Autodesk Fusion 360 part; units mm, degrees
sketch "Sketch1" plane through (0, 0, 0) normal (0, 1, 0) x (1, 0, 0)
  line L0 (-21.4929, -3.9767) -> (-14.25, -3.9767)
  arc A0 (14.25, 0) -> (-14.25, 0) centre (0, 0) ccw
  line L1 (-21.4929, -3.9767) -> (-21.4929, 15.251)
  line L2 (21.5026, 15.251) -> (-21.4929, 15.251)
  circle A1 centre (-17.5048, 0.0114) radius 2.1
  line L3 (21.5026, -4.0254) -> (14.25, -4.0217)
  circle A2 centre (17.4952, -0.0012) radius 2.1
  line L4 (21.5026, -4.0254) -> (21.5026, 15.251)
  line L5 (-21.4929, 11.251) -> (-8.7451, 11.251)
  line L6 (8.7451, 11.251) -> (21.5026, 11.251)
  line L7 (-14.25, -3.9767) -> (-14.25, 0)
  line L8 (14.25, 0) -> (14.25, -4.0217)
  dimension "d1" = 28.5
  dimension "d4" = 4.2
  dimension "d14" = 4
  dimension "d33" = 35
  dimension "d34" = 4.2
extrude "Extrude1" add sketch "Sketch1" along normal blind 5 from surface at 1
extrude "Extrude3" add sketch "Sketch1" along normal blind 20 contours A0 L1 L2 L4 L5 L6
sketch "Sketch4" plane through (0, 0, -15.251) normal (0, 0, -1) x (1, 0, 0)
  line L0 (-21.4929, 0) -> (-21.4929, -20)
  line L1 (-21.4929, -20) -> (21.5026, -20)
  line L2 (21.5026, -20) -> (21.5026, 0)
  line L3 (-21.4929, 0) -> (-21.4929, -20)
  line L4 (-21.4929, -20) -> (21.5026, -20)
  line L5 (21.5026, -20) -> (21.5026, 0)
  line L6 (21.5026, 0) -> (-21.4929, 0)
  circle A0 centre (-14.9976, -10) radius 1.6
  line L7 (0.0024, 3.9978) -> (0.0024, -22.1306)
  circle A1 centre (15.0024, -10) radius 1.6
  dimension "d50" = 3.2
  dimension "d51" = 10
  dimension "d52" = 15
extrude "Extrude8" cut sketch "Sketch4" along normal blind -8 and the other way blind -2 contours A0 | A1
chamfer "Chamfer1" distance 1 angle 45 4 edges at (-15.119, 1, -11.251) (15.1239, 1, -11.251) (-15.119, 6, -11.251) (15.1239, 6, -11.251)
fillet "Fillet1" radius 14 2 edges at (-21.4929, 20, -13.251) (21.5026, 20, -13.251)
equation "d34 = d4"
Can you work these out from the model? Positions are in its coordinate system, mm. A direction names the side the tool comes from. Round coordinates to 2 decimals unless told otherwise and drop trailing zeros. Loops run counter-clockwise (first coordinate to the right, second up) from the corner with the lowest first, then second, coordinate; pieces in that order, holes last.
Item 1: Suppose I cut it at D-D, the plane y = 5.5. Write out the boundary of the cut face in (x, z).
Item 2: Suppose I cut it at C-C, the plane y = 10. Write out the boundary of the cut face in (x, z), then the cut area to 3 significant figures.
Item 3: If we mould it in two halves opening along X, with no side actions, what happens to faces 1 (the cylindrical face through (-0.313, 7.638, -14.247)), 2 (the cylindrical face through (-14.26, 11.42, -13.28)), 3 (the flat face through (21.503, 4, -5)), 4 (the flat face through (-17, 6, -5))? For each: +X half, -X half, draft (parallel to the pull), parting line (faces both ways), or undercut.
Item 4: Will these pins go through, and if not, where does the flat tip stop? pin 1 Ø1.9 at (x, y) = (-15, 10) entering from +Z; pin 2 Ø6 at (x, z) = (-15.5, 1.5) entering from +Y; pin 3 Ø4 at (x, y) = (-14, 12) entering from +Z; pin 4 Ø6 at (x, z) = (15, -6) entering from -Y.
Item 5: Which directions (+Z, -Z, +X, -X, +Y, -Y) give clear straight access to the entire face, cutting with the end or side of a thin tool? Please do faces 5 (the flat face through (-17, 1, -5)), 6 (the flat face through (-14, 12, -11.251)), 7 (the flat face through (-14.25, 3, 2)).
Item 6: Please list where these lines run through material, in increasing order: L1, parallel to X at y = 11, z = -13.25; L2, parallel to X at y = 10, z = -12.8; L3, parallel to Z at x = -13, y = 8.25.
Item 7: Suppose I cut it at A-A, the plane x = 16. State how many separate pieces and enclosed holes the cut face has, then the cut area to 3 significant figures.
Item 8: Suppose I cut it at B-B, the plane z = -7.5. Write out the boundary of the cut face in (x, y), then the cut area to 3 significant figures.
Reported:
1. outline: (-21.49, -15.25) - (21.5, -15.25) - (21.5, 4.03) - (14.25, 4.02) - (14.25, 0) arc R14.25 cw to (-14.25, 0) - (-14.25, 3.98) - (-21.49, 3.98) - close; hole circle Ø4.2 at (-17.5, -0.01); hole circle Ø4.2 at (17.5, 0)
2. outline: (-20.91, -15.25) - (-16.6, -15.25) - (-16.6, -11.25) - (-20.91, -11.25) - close; (-13.4, -15.25) - (13.4, -15.25) - (13.4, -11.25) - (8.75, -11.25) arc R14.25 cw to (-8.75, -11.25) - (-13.4, -11.25) - close; (16.6, -15.25) - (20.92, -15.25) - (20.92, -11.25) - (16.6, -11.25) - close
2. area: 106 mm2
3. face 1: undercut
3. face 2: undercut
3. face 3: +X half
3. face 4: draft
4. pin 1: passes through
4. pin 2: stops at y = 6
4. pin 3: stops at z = -11.25
4. pin 4: stops at y = 1
5. face 5: +Z, +X, -X, -Y
5. face 6: +Z, +X, -X, +Y
5. face 7: +Z, +Y, -Y
6. L1: x = -20.57 to -16.25, -13.75 to -5.24, 5.24 to 13.75, 16.25 to 20.58
6. L2: x = -20.91 to -16.6, -13.4 to -6.26, 6.26 to 13.4, 16.6 to 20.92
6. L3: z = -15.25 to -11.25
7. separate pieces: 3
7. enclosed holes: 0
7. area: 121 mm2
8. outline: (-21.49, 1) - (-12.12, 1) - (-12.12, 6) - (-21.49, 6) - close; (12.12, 1) - (21.5, 1) - (21.5, 6) - (12.12, 6) - close
8. area: 93.8 mm2
